from build123d import *

# Parameters (mm, degrees)
SKETCH1_W           = 10
SKETCH1_H           = 3
BOSS_EXTRUDE1_DEPTH = 5
FILLET2_R           = 0.5


with BuildPart() as part:
    # Sketch1 → Boss-Extrude1 (new body)
    with BuildSketch(Plane.XY):
        Polygon((-7, -4), (7, -4), (7, 4), (1.5, 4), (1.5, 5.55), (7, 5.55), (7, 7.05), (-7, 7.05), (-7, 5.55), (-1.5, 5.55), (-1.5, 4), (-7, 4), align=None)
        Rectangle(SKETCH1_W, SKETCH1_H, mode=Mode.SUBTRACT)
    extrude(amount=BOSS_EXTRUDE1_DEPTH)

    # Fillet2
    fillet2_edges = [part.edges().sort_by_distance(p)[0] for p in [
        (-7, 4, 2.5),
        (-1.5, 4, 2.5),
        (-1.5, 5.55, 2.5),
        (-7, 5.55, 2.5),
        (-7, 7.05, 2.5),
        (7, 7.05, 2.5),
        (7, 5.55, 2.5),
        (1.5, 5.55, 2.5),
        (1.5, 4, 2.5),
        (7, 4, 2.5),
        (7, -4, 2.5),
        (-7, -4, 2.5),
        (-5, 1.5, 2.5),
        (-5, -1.5, 2.5),
        (5, -1.5, 2.5),
        (5, 1.5, 2.5),
    ]]
    fillet(fillet2_edges, radius=FILLET2_R)


solid = part.part
Source: CAD feature listing. Evaluate the final solid. Frame: model axes, mm. A direction names the side the tool comes from. Coordinates: 2 decimals unless noted, no trailing zeros. Loops run counter-clockwise (first coordinate to the right, second up) from the corner with the lowest first, then second, coordinate; pieces in that order, holes last. Notation, with made-up numbers: (41, 29) -> (73, 29) arc R17 cw to (73, 57) -> close; hole circle Ø7 at (63.25, -23). An arc over 180 degrees is marked (long way). Answer in a Markdown table with one row per item. Add a question column.
Q1. Section B-B on y = 0. Return the cut outline in (x, z), and give its area (3 significant figures).
Q2. Section C-C on x = 6.25. Return the cut outline in (y, z), and give its area (3 significant figures).
Q3. Section A-A on x = -3.5. Return the cut outline in (y, z), and give its area (3 significant figures).
Q4. Pull-direction query (X, two-part tool) for faces 5 (the face through (-7, 0, 2)), 6 (the face through (0, -4, 2)), 7 (the face through (0, -1.5, 2)); classes: pulls with the +X half, pulls with the -X half, needs draft (parallel to the pull), parting line crosses it, or undercut.
Q5. Ray query, line 1 along Y through (x, z) = (4.5, 1.9); line 2 along Y through (x, z) = (-1.25, 0.6). Return the intervals inside material, ascending.
Q6. Reachability of faces 1 (the face through (4, 4, 2)), 2 (the face through (0, 2, 5)), 3 (the face through (-4, 4, 2)), 4 (the face through (-5, 0, 2)) from +Z, -Z, +X, -X, +Y, -Y: full face, straight path, thin tool, end or side. Return the list, or none.
Q7. Contact query for a flat-ended pin moving along its axis: pin 1 Ø2 at (y, z) = (5, 0.5) entering from +X. Output: stop coordinate, or through.
Computed values:
| question | item | result |
|---|---|---|
| 1 | outline | (-7, 0) -> (-5, 0) -> (-5, 5) -> (-7, 5) -> close; (5, 0) -> (7, 0) -> (7, 5) -> (5, 5) -> close |
| 1 | area | 20.0 mm^2 |
| 2 | outline | (-4, 0) -> (4, 0) -> (4, 5) -> (-4, 5) -> close; (5.55, 0) -> (7.05, 0) -> (7.05, 5) -> (5.55, 5) -> close |
| 2 | area | 47.5 mm^2 |
| 3 | outline | (-4, 0) -> (-1.5, 0) -> (-1.5, 5) -> (-4, 5) -> close; (1.5, 0) -> (4, 0) -> (4, 5) -> (1.5, 5) -> close; (5.55, 0) -> (7.05, 0) -> (7.05, 5) -> (5.55, 5) -> close |
| 3 | area | 32.5 mm^2 |
| 4 | face 5 | pulls with the -X half |
| 4 | face 6 | needs draft |
| 4 | face 7 | undercut |
| 5 | line 1 | y = -4 to -1.5, 1.5 to 4, 5.55 to 7.05 |
| 5 | line 2 | y = -4 to -1.5, 1.5 to 7.05 |
| 6 | face 1 | +Z, -Z, +X |
| 6 | face 2 | +Z, +X, -X, +Y, -Y |
| 6 | face 3 | +Z, -Z, -X |
| 6 | face 4 | +Z, -Z |
| 7 | pin 1 | stops at x = 7 |
